```python
from build123d import *

# Parameters (mm, degrees)
BOSS_EXTRUDE1_DEPTH = 1.6
CUT_EXTRUDE1_START  = 1.6
SKETCH2_R           = 1.25
CUT_EXTRUDE1_DEPTH  = 2.5
FILLET1_R           = 5


with BuildPart() as part:
    # Sketch1 → Boss-Extrude1 (new body)
    with BuildSketch(Plane(origin=(0, 0, 0), x_dir=(1, 0, 0), z_dir=(0, 1, 0))):
        Polygon((17.7, 36), (-17.7, 36), (-30, 7.2), (-30, -36), (30, -36), (30, 7.2), align=None)
    extrude(amount=BOSS_EXTRUDE1_DEPTH)

    # Sketch2 → Cut-Extrude1 (cut)
    with BuildSketch(Plane(origin=(0, 0, 0), x_dir=(1, 0, 0), z_dir=(0, 1, 0)).offset(CUT_EXTRUDE1_START)):
        with Locations((-27, -24)):
            Circle(SKETCH2_R)
        with Locations((27, -24)):
            Circle(SKETCH2_R)
        with Locations((26, 8)):
            Circle(SKETCH2_R)
        with Locations((-26, 8)):
            Circle(SKETCH2_R)
        with Locations((-22, -31)):
            Circle(SKETCH2_R)
        with Locations((22, -31)):
            Circle(SKETCH2_R)
    extrude(amount=-CUT_EXTRUDE1_DEPTH, mode=Mode.SUBTRACT)

    # Fillet1
    fillet1_edges = [part.edges().sort_by_distance(p)[0] for p in [
        (30, 0.8, -7.2),
        (30, 0.8, 36),
        (-30, 0.8, 36),
        (-30, 0.8, -7.2),
        (-17.7, 0.8, -36),
        (17.7, 0.8, -36),
    ]]
    fillet(fillet1_edges, radius=FILLET1_R)


solid = part.part
```
CAD build for the part. Positions are in the model's coordinates, mm. Round coordinates to 2 decimals unless told otherwise and drop trailing zeros. Order: outer loops, then holes, each group sorted by start corner. A loop starts at its lowest first (then second) coordinate and runs counter-clockwise, first axis right, second up. Notation, with made-up numbers: (19, -16.5) - (78, -16.5) arc R30 cw to (78, 12.5) - close; hole circle Ø6 at (-10.5, 72.5). An arc over 180 degrees is marked (long way). Answer as CSV lines item,"result". Start each with the question number.
1. Saw through at A-A, the plane z = 24. Write the cut outline in (x, y), and give its area (3 significant figures).
2. Saw through at B-B, the plane x = 22. Write the cut outline in (y, z).
3. Saw through at C-C, the plane y = 0.3. Write the cut outline in (x, z).
4. Drill centre lines: L1, parallel to X at y = 0.75, z = 24; L2, parallel to X at y = 0.45, z = 31; L3, parallel to Z at x = 27, y = 1.1. Where is each one in solid material? Low to high. Write a range as [from, to].
5. Pull direction X, two halves, no side cores. Call faces 1 (the face through (24.37, 0.79, -20.38)), 2 (the face through (0, 1, 36)), 3 (the face through (-25.845, 0.811, 24.479)), 4 (the face through (-17.119, 0.811, -35.195)): +X half, -X half, draft (parallel to the pull), parting line (faces both ways), or undercut.
Model answer:
1,outline,"(-30, 0) - (-28.25, 0) - (-28.25, 1.6) - (-30, 1.6) - close; (-25.75, 0) - (25.75, 0) - (25.75, 1.6) - (-25.75, 1.6) - close; (28.25, 0) - (30, 0) - (30, 1.6) - (28.25, 1.6) - close"
1,area,"88.0 mm²"
2,outline,"(0, -25.93) - (1.6, -25.93) - (1.6, 29.75) - (0, 29.75) - close; (0, 32.25) - (1.6, 32.25) - (1.6, 36) - (0, 36) - close"
3,outline,"(-30, -6.18) arc R5 ccw to (-29.6, -8.14) - (-19, -32.96) arc R5 ccw to (-14.4, -36) - (14.4, -36) arc R5 ccw to (19, -32.96) - (29.6, -8.14) arc R5 ccw to (30, -6.18) - (30, 31) arc R5 ccw to (25, 36) - (-25, 36) arc R5 ccw to (-30, 31) - close; hole circle Ø2.5 at (-27, 24); hole circle Ø2.5 at (-26, -8); hole circle Ø2.5 at (-22, 31); hole circle Ø2.5 at (22, 31); hole circle Ø2.5 at (26, -8); hole circle Ø2.5 at (27, 24)"
4,L1,"x = [-30, -28.25], [-25.75, 25.75], [28.25, 30]"
4,L2,"x = [-30, -23.25], [-20.75, 20.75], [23.25, 30]"
4,L3,"z = [-14.22, -8.75], [-7.25, 22.75], [25.25, 35.58]"
5,face 1,"+X half"
5,face 2,"draft"
5,face 3,"undercut"
5,face 4,"-X half"
